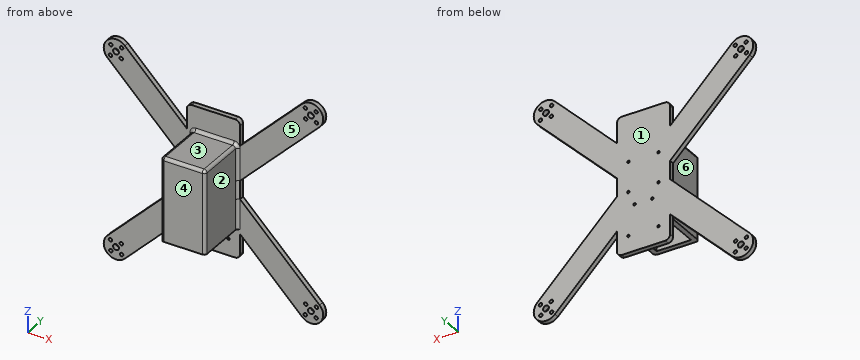
```python
from build123d import *

# Parameters (mm, degrees)
BOSS_EXTRUDE1_DEPTH       = 5
CUT_EXTRUDE1_REACH        = 159.757
SKETCH3_R                 = 3
SKETCH3_R_2               = 1.75
MIRROR2_COPY_1_REACH      = 159.757
MIRROR2_COPY_1_SKETCH_R   = 3
MIRROR2_COPY_1_SKETCH_R_2 = 1.75
M3X0_5_TAPPED_HOLE1_D     = 2.5
BOSS_EXTRUDE2_DEPTH       = 47
SKETCH7_W                 = 45
SKETCH7_H                 = 85
BOSS_EXTRUDE3_DEPTH       = 5
FILLET1_R                 = 5
FILLET2_R                 = 3


with BuildPart() as part:
    # Sketch2 → Boss-Extrude1 (new body)
    with BuildSketch(Plane(origin=(0, 0, 0), x_dir=(1, 0, 0), z_dir=(0, 1, 0))):
        with BuildLine():
            Line((-27, 70), (27, 70))
            Line((27, 70), (27, 44.67766953))
            Line((27, 44.67766953), (90.156114601, 107.833784131))
            ThreePointArc((90.156114601, 107.833784131), (107.833784131, 107.833784131), (107.833784131, 90.156114601))
            Line((107.833784131, 90.156114601), (27, 9.32233047))
            Line((27, 9.32233047), (27, -9.32233047))
            Line((27, -9.32233047), (107.833784131, -90.156114601))
            ThreePointArc((107.833784131, -90.156114601), (107.833784131, -107.833784131), (90.156114601, -107.833784131))
            Line((90.156114601, -107.833784131), (27, -44.67766953))
            Line((27, -44.67766953), (27, -70))
            Line((27, -70), (-27, -70))
            Line((-27, -70), (-27, -44.67766953))
            Line((-27, -44.67766953), (-90.156114601, -107.833784131))
            ThreePointArc((-90.156114601, -107.833784131), (-107.833784131, -107.833784131), (-107.833784131, -90.156114601))
            Line((-107.833784131, -90.156114601), (-27, -9.32233047))
            Line((-27, -9.32233047), (-27, 9.32233047))
            Line((-27, 9.32233047), (-107.833784131, 90.156114601))
            ThreePointArc((-107.833784131, 90.156114601), (-107.833784131, 107.833784131), (-90.156114601, 107.833784131))
            Line((-90.156114601, 107.833784131), (-27, 44.67766953))
            Line((-27, 44.67766953), (-27, 70))
        make_face()
    extrude(amount=BOSS_EXTRUDE1_DEPTH)

    # Sketch3 → Cut-Extrude1 (cut, up to next)
    with BuildSketch(Plane(origin=(0, 5, 0), x_dir=(1, 0, 0), z_dir=(0, 1, 0)), mode=Mode.PRIVATE) as cut_extrude1_sk1:
        with Locations(Location((-98.994949366, -98.994949366, 0), (0, 0, 270))):
            Circle(SKETCH3_R)
    cut_extrude1_tool1 = extrude(cut_extrude1_sk1.sketch, amount=-CUT_EXTRUDE1_REACH, mode=Mode.PRIVATE) & part.part
    # Sketch3 → Cut-Extrude1 (cut, up to next)
    with BuildSketch(Plane(origin=(0, 5, 0), x_dir=(1, 0, 0), z_dir=(0, 1, 0)), mode=Mode.PRIVATE) as cut_extrude1_sk2:
        with Locations(Location((-104.298250225, -104.298250225, 0), (0, 0, 270))):
            Circle(SKETCH3_R_2)
    cut_extrude1_tool2 = extrude(cut_extrude1_sk2.sketch, amount=-CUT_EXTRUDE1_REACH, mode=Mode.PRIVATE) & part.part
    # Sketch3 → Cut-Extrude1 (cut, up to next)
    with BuildSketch(Plane(origin=(0, 5, 0), x_dir=(1, 0, 0), z_dir=(0, 1, 0)), mode=Mode.PRIVATE) as cut_extrude1_sk3:
        with Locations(Location((-93.338095117, -104.651803616, 0), (0, 0, 270))):
            Circle(SKETCH3_R_2)
    cut_extrude1_tool3 = extrude(cut_extrude1_sk3.sketch, amount=-CUT_EXTRUDE1_REACH, mode=Mode.PRIVATE) & part.part
    # Sketch3 → Cut-Extrude1 (cut, up to next)
    with BuildSketch(Plane(origin=(0, 5, 0), x_dir=(1, 0, 0), z_dir=(0, 1, 0)), mode=Mode.PRIVATE) as cut_extrude1_sk4:
        with Locations(Location((-104.651803616, -93.338095117, 0), (0, 0, 270))):
            Circle(SKETCH3_R_2)
    cut_extrude1_tool4 = extrude(cut_extrude1_sk4.sketch, amount=-CUT_EXTRUDE1_REACH, mode=Mode.PRIVATE) & part.part
    # Sketch3 → Cut-Extrude1 (cut, up to next)
    with BuildSketch(Plane(origin=(0, 5, 0), x_dir=(1, 0, 0), z_dir=(0, 1, 0)), mode=Mode.PRIVATE) as cut_extrude1_sk5:
        with Locations(Location((-93.691648507, -93.691648507, 0), (0, 0, 270))):
            Circle(SKETCH3_R_2)
    cut_extrude1_tool5 = extrude(cut_extrude1_sk5.sketch, amount=-CUT_EXTRUDE1_REACH, mode=Mode.PRIVATE) & part.part
    cut_extrude1_1 = cut_extrude1_tool1.solids().sort_by_distance((-98.994949, 5, 98.994949))[0]
    add(cut_extrude1_1, mode=Mode.SUBTRACT)
    cut_extrude1_2 = cut_extrude1_tool2.solids().sort_by_distance((-104.29825, 5, 104.29825))[0]
    add(cut_extrude1_2, mode=Mode.SUBTRACT)
    cut_extrude1_3 = cut_extrude1_tool3.solids().sort_by_distance((-93.338095, 5, 104.651804))[0]
    add(cut_extrude1_3, mode=Mode.SUBTRACT)
    cut_extrude1_4 = cut_extrude1_tool4.solids().sort_by_distance((-104.651804, 5, 93.338095))[0]
    add(cut_extrude1_4, mode=Mode.SUBTRACT)
    cut_extrude1_5 = cut_extrude1_tool5.solids().sort_by_distance((-93.691649, 5, 93.691649))[0]
    add(cut_extrude1_5, mode=Mode.SUBTRACT)
    cut_extrude1 = cut_extrude1_1 + cut_extrude1_2 + cut_extrude1_3 + cut_extrude1_4 + cut_extrude1_5  # Cut-Extrude1 as one shape, for the pattern or mirror that repeats it

    # Mirror1: Cut-Extrude1 across plane
    add(cut_extrude1.mirror(Plane(origin=(0, 0, 0), x_dir=(0, 0, 1), z_dir=(1, 0, 0))), mode=Mode.SUBTRACT)

    # Mirror2: Cut-Extrude1 across plane
    add(cut_extrude1.mirror(Plane.XY), mode=Mode.SUBTRACT)

    # Mirror2 copy 1 sketch → Mirror2 copy 1 (cut, up to next)
    with BuildSketch(Plane(origin=(0, 5, 0), x_dir=(-1, 0, 0), z_dir=(0, 1, 0)), mode=Mode.PRIVATE) as mirror2_copy_1_sk1:
        with Locations(Location((-98.994949366, -98.994949366, 0), (0, 0, 270))):
            Circle(MIRROR2_COPY_1_SKETCH_R)
    mirror2_copy_1_tool1 = extrude(mirror2_copy_1_sk1.sketch, amount=-MIRROR2_COPY_1_REACH, mode=Mode.PRIVATE) & part.part
    # Mirror2 copy 1 sketch → Mirror2 copy 1 (cut, up to next)
    with BuildSketch(Plane(origin=(0, 5, 0), x_dir=(-1, 0, 0), z_dir=(0, 1, 0)), mode=Mode.PRIVATE) as mirror2_copy_1_sk2:
        with Locations(Location((-104.298250225, -104.298250225, 0), (0, 0, 270))):
            Circle(MIRROR2_COPY_1_SKETCH_R_2)
    mirror2_copy_1_tool2 = extrude(mirror2_copy_1_sk2.sketch, amount=-MIRROR2_COPY_1_REACH, mode=Mode.PRIVATE) & part.part
    # Mirror2 copy 1 sketch → Mirror2 copy 1 (cut, up to next)
    with BuildSketch(Plane(origin=(0, 5, 0), x_dir=(-1, 0, 0), z_dir=(0, 1, 0)), mode=Mode.PRIVATE) as mirror2_copy_1_sk3:
        with Locations(Location((-93.338095117, -104.651803616, 0), (0, 0, 270))):
            Circle(MIRROR2_COPY_1_SKETCH_R_2)
    mirror2_copy_1_tool3 = extrude(mirror2_copy_1_sk3.sketch, amount=-MIRROR2_COPY_1_REACH, mode=Mode.PRIVATE) & part.part
    # Mirror2 copy 1 sketch → Mirror2 copy 1 (cut, up to next)
    with BuildSketch(Plane(origin=(0, 5, 0), x_dir=(-1, 0, 0), z_dir=(0, 1, 0)), mode=Mode.PRIVATE) as mirror2_copy_1_sk4:
        with Locations(Location((-104.651803616, -93.338095117, 0), (0, 0, 270))):
            Circle(MIRROR2_COPY_1_SKETCH_R_2)
    mirror2_copy_1_tool4 = extrude(mirror2_copy_1_sk4.sketch, amount=-MIRROR2_COPY_1_REACH, mode=Mode.PRIVATE) & part.part
    # Mirror2 copy 1 sketch → Mirror2 copy 1 (cut, up to next)
    with BuildSketch(Plane(origin=(0, 5, 0), x_dir=(-1, 0, 0), z_dir=(0, 1, 0)), mode=Mode.PRIVATE) as mirror2_copy_1_sk5:
        with Locations(Location((-93.691648507, -93.691648507, 0), (0, 0, 270))):
            Circle(MIRROR2_COPY_1_SKETCH_R_2)
    mirror2_copy_1_tool5 = extrude(mirror2_copy_1_sk5.sketch, amount=-MIRROR2_COPY_1_REACH, mode=Mode.PRIVATE) & part.part
    add(mirror2_copy_1_tool1.solids().sort_by_distance((98.994949, 5, -98.994949))[0], mode=Mode.SUBTRACT)
    add(mirror2_copy_1_tool2.solids().sort_by_distance((104.29825, 5, -104.29825))[0], mode=Mode.SUBTRACT)
    add(mirror2_copy_1_tool3.solids().sort_by_distance((93.338095, 5, -104.651804))[0], mode=Mode.SUBTRACT)
    add(mirror2_copy_1_tool4.solids().sort_by_distance((104.651804, 5, -93.338095))[0], mode=Mode.SUBTRACT)
    add(mirror2_copy_1_tool5.solids().sort_by_distance((93.691649, 5, -93.691649))[0], mode=Mode.SUBTRACT)

    # M3x0.5 Tapped Hole1 (through all)
    with Locations(Plane(origin=(0, 5, 0), x_dir=(1, 0, 0), z_dir=(0, 1, 0))):
        with Locations((-15.25, -22), (15.25, -22), (-15.25, 8.5), (15.25, 8.5), (-9, 23), (9, 23), (-15.25, 53), (15.25, 53)):
            Hole(M3X0_5_TAPPED_HOLE1_D / 2)

    # Sketch6 → Boss-Extrude2 (add)
    with BuildSketch(Plane.XZ):
        Polygon((-15.881026332, -40), (-20.881026332, -40), (-20.881026332, 45), (24.118973668, 45), (24.118973668, -40), (19.118973668, -40), (19.118973668, 40), (-15.881026332, 40), align=None)
    extrude(amount=BOSS_EXTRUDE2_DEPTH)

    # Sketch7 → Boss-Extrude3 (add)
    with BuildSketch(Plane.XZ.offset(47)):
        with Locations((1.618973668, 2.5)):
            Rectangle(SKETCH7_W, SKETCH7_H)
    extrude(amount=BOSS_EXTRUDE3_DEPTH)

    # Fillet1
    fillet1_edges = [part.edges().sort_by_distance(p)[0] for p in [
        (27, 2.5, 70),
        (-27, 2.5, 70),
        (-27, 2.5, -70),
        (27, 2.5, -70),
    ]]
    fillet(fillet1_edges, radius=FILLET1_R)

    # Fillet2
    fillet2_edges = [part.edges().sort_by_distance(p)[0] for p in [
        (-20.881026332, 0, 2.5),
        (-20.881026332, -26, 45),
        (24.118973668, 0, 2.5),
        (1.618973668, 0, 45),
        (24.118973668, -26, 45),
        (-20.881026332, -52, 2.5),
        (24.118973668, -52, 2.5),
        (1.618973668, -52, 45),
    ]]
    fillet(fillet2_edges, radius=FILLET2_R)


solid = part.part
```
Could you check a few things on this model? Use its own coordinates, in mm. Face numbers are marked on the shaded views. A direction names the side the tool comes from. Coordinates: 2 decimals unless noted, no trailing zeros. Write each loop counter-clockwise with the first axis right and the second up, starting at its lowest first coordinate (ties: lowest second). Pieces come first, ordered by that corner, then holes. Notation, with made-up numbers: M -37.75,44.25 L -30.75,44.25 A26 cw -30.75,80.25 Z; hole C 55,38.25 d9. An arc over 180 degrees is marked long. Answer as CSV lines item,"result". Start each with the question number.
1) Please list where these lines run through material, in increasing order: line 1 (X direction, y = -21, z = 23); line 2 (Y direction, x = 8.5, z = -19.5); line 3 (Z direction, x = -5, y = -21). Write a range as from..to.
2) For the marked faces 1, 2 and 3, which set-ups out of +Z, -Z, +X, -X, +Y, -Y let a thin tool reach every point of the face, with its end or its side?
3) I want a section at B-B, the plane x = -53. Please give me the cut outline in (y, z).
4) We'd pull the mould along X, two halves only. Please class the marked faces 4, 5 and 6: +X half, -X half, draft (parallel to the pull), parting line (faces both ways), or undercut.
5) For P1, Ø2, axis at x = -15.25, z = -8.5, coming from the +Y side; P2, Ø5.5, axis at y = 1.5, z = 3, coming from the -X side; P3, Ø1, axis at x = 16, z = 50.5, coming from the -Y side, each with a flat end and sliding along its axis, tell me the tip position at first contact or that it passes through.
6) I want a section at A-A, the plane y = -27. Please give me the cut outline in (x, z), and give its area (3 significant figures).
Data:
1,line 1,"x = -20.88..-15.88, 19.12..24.12"
1,line 2,"y = -52..-47, 0..5"
1,line 3,"z = 40..45"
2,face 1,"+Z, -Z, +X, -X, +Y"
2,face 2,"+Z, -Z, +X, -Y"
2,face 3,"+Z, +X, -X, -Y"
3,outline,"M 0,-70.68 L 5,-70.68 L 5,-35.32 L 0,-35.32 Z; M 0,35.32 L 5,35.32 L 5,70.68 L 0,70.68 Z"
4,face 4,"draft"
4,face 5,"undercut"
4,face 6,"-X half"
5,P1,"stops at y = 0"
5,P2,"stops at x = -27"
5,P3,"stops at y = 0"
6,outline,"M -20.88,-40 L -15.88,-40 L -15.88,40 L 19.12,40 L 19.12,-40 L 24.12,-40 L 24.12,42 A3 ccw 21.12,45 L -17.88,45 A3 ccw -20.88,42 Z"
6,area,"1,020 mm^2"
